Geometry: final body of the model. Coordinates: model frame, mm. A direction names the side the tool comes from. Round coordinates to 2 decimals unless told otherwise and drop trailing zeros. Order: outer loops, then holes, each group sorted by start corner. A loop starts at its lowest first (then second) coordinate and runs counter-clockwise, first axis right, second up. Notation, with made-up numbers: M 22,65 L 67,65 A18 cw 67,83 Z; hole C 33,2.25 d5. An arc over 180 degrees is marked long. Return JSON: item names as keys, results as strings. Group by question number.
Q1. Ray query, probe 1 along Z at (x, y) = (1.8, 0); probe 2 along X at (y, z) = (4, 11.5); probe 3 along Z at (x, y) = (2.25, -1). Return the intervals inside material, ascending.
Q2. Access query for faces 4 (the face through (24.33, -3, -3)), 5 (the face through (4.83, 6.89, -3.33)). Directions: +Z, -Z, +X, -X, +Y, -Y. A direction counts if a zero-diameter tool reaches every point of the face in a straight line with its end or side. Return the directions, or none.
Q3. Cut plane A-A on y = -12. Output: boundary loops of the cut face in (x, z).
Q4. Cut plane C-C on x = 12.5. Output: boundary loops of the cut face in (y, z), and give its area (3 significant figures).
Q5. Mould query, pull axis Z, two halves, no side actions, for faces 1 (the face through (11.995, 3.146, 2.471)), 2 (the face through (0, 3, -3)), 3 (the face through (2.38, -3.47, 15.62)). Classes: released by +Z, released by -Z, zero draft, split by the parting line, or undercut.
Q6. Contact query for flat-ended pins moving along their axis: pin 1 (4 mm diameter, centred on y = 12, z = 0, fed in from +X); pin 2 (12 mm diameter, centred on x = 5.5, y = -8.5, fed in from -Z); pin 3 (6 mm diameter, centred on y = -6, z = 6.5, fed in from -X); pin 4 (5 mm diameter, centred on x = 14.5, y = -5.5, fed in from +Z). Output: stop coordinate, or through.
Autodesk Inventor part; units mm, degrees
ref_plane "YZ Plane" through (0, 0, 0) normal (1, 0, 0) x (0, 1, 0)
ref_plane "XZ Plane" through (0, 0, 0) normal (0, 1, 0) x (-1, 0, 0)
ref_plane "XY Plane" through (0, 0, 0) normal (0, 0, 1) x (1, 0, 0)
sketch "Sketch1" plane through (0, 0, 0) normal (1, 0, 0) x (0, 1, 0)
  circle A0 centre (0, 0) radius 16
  circle A1 centre (-12, 0) radius 1.75
  circle A2 centre (0, -12) radius 1.75
  circle A3 centre (12, 0) radius 1.75
  circle A4 centre (0, 12) radius 1.75
  circle A5 centre (0, 0) radius 7.5
  circle A6 centre (0, 0) radius 4
  dimension "d0" = 32
  dimension "d1" = 3.5
  dimension "d4" = 360
  dimension "d6" = 24
  dimension "d7" = 15
  dimension "d8" = 8
  dimension "d14" = 12
extrude "Extrusion1" add sketch "Sketch1" along normal blind 4.83 contours A0 | A5
sketch "Sketch2" plane through (4.83, 0, 0) normal (1, 0, 0) x (0, 0, -1)
  circle A0 centre (0, 0) radius 4
  circle A1 centre (0, 0) radius 7.5
  point P0 (0, 0)
  dimension "d11" = 15
extrude "Extrusion2" add sketch "Sketch2" along normal blind 19.5
properties part number "linear bearing"
Result sheet:
{
 "1": {"probe 1": "z = -16 to -13.75, -10.25 to -4, 4 to 10.25, 13.75 to 16", "probe 2": "x = 0 to 4.83", "probe 3": "z = -15.97 to -13.44, -10.56 to -3.87, 3.87 to 10.56, 13.44 to 15.97"},
 "2": {"face 4": "+Z, -Z, +X, +Y, -Y", "face 5": "+X"},
 "3": {"outline": "M 0,-10.58 L 4.83,-10.58 L 4.83,-1.75 L 0,-1.75 Z; M 0,1.75 L 4.83,1.75 L 4.83,10.58 L 0,10.58 Z"},
 "4": {"outline": "C 0,0 d15; hole C 0,0 d8", "area": "126 mm²"},
 "5": {"face 1": "undercut", "face 2": "zero draft", "face 3": "split by the parting line"},
 "6": {"pin 1": "stops at x = 4.83", "pin 2": "stops at z = -15.8", "pin 3": "stops at x = 0", "pin 4": "stops at z = 6.87"}
}
